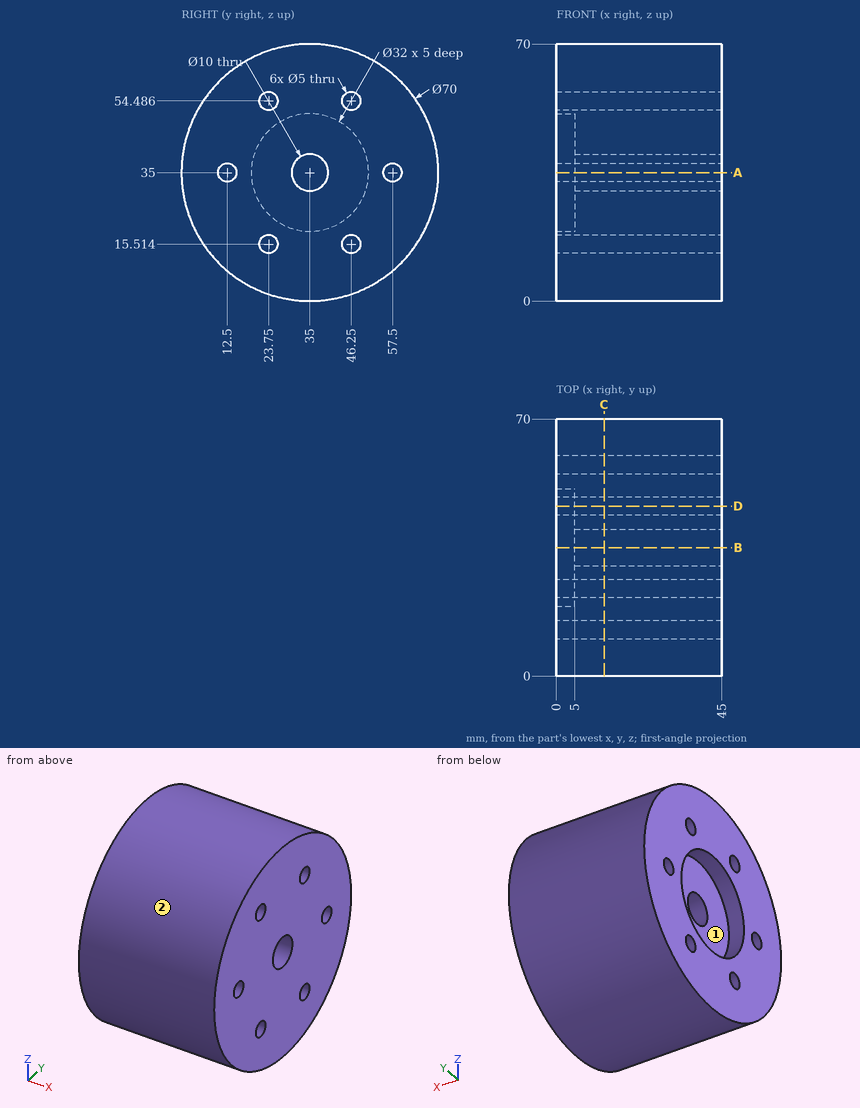
Can you work these out from the drawing? Everything is in mm from the part's minimum corner. A direction names the side the tool comes from. Give positions to 0.01 mm unless a question says otherwise; leave off trailing zeros. Loops run counter-clockwise (first coordinate to the right, second up) from the corner with the lowest first, then second, coordinate; pieces in that order, holes last. Notation, with made-up numbers: (7, 39.5) - (44, 39.5) arc R12 cw to (44, 49.5) - close; hole circle Ø1 at (19.25, -31). An arc over 180 degrees is marked (long way). Use one line per item in the form item = value.
1. I'm going to push flat-ended pins straight in: pin 1 Ø4.5 at (y, z) = (23.75, 54.49) entering from -X; pin 2 Ø1 at (y, z) = (25.5, 46.5) entering from -X; pin 3 Ø6 at (x, y) = (5.5, 59.5) entering from -Z; pin 4 Ø1 at (x, z) = (5.5, 40) entering from +Y. Where does each tip first touch, or does it pass through?
Response values:
pin_1 = through
pin_2 = 5
pin_3 = 7.38
pin_4 = 69.71
2. I want a section at D-D (y = 46.25). Please give me the cut outline in (x, z) (1 decimal), and give its area (3 significant figures).
Response values:
outline = (0, 1.9) - (45, 1.9) - (45, 13) - (0, 13) - close; (0, 18) - (45, 18) - (45, 52) - (0, 52) - (0, 46.4) - (5, 46.4) - (5, 23.6) - (0, 23.6) - close; (0, 57) - (45, 57) - (45, 68.1) - (0, 68.1) - close
area = 2,420 mm²
3. I want a section at C-C (x = 13). Give the number of separate pieces and of enclosed holes in the cut face, and give its area (3 significant figures).
Response values:
separate_pieces = 1
enclosed_holes = 7
area = 3,650 mm²
4. I need wall thicknesses on probe 1 along Y at (x, z) = (24, 35); probe 2 along Z at (x, y) = (9, 23); probe 3 along Z at (x, y) = (19, 23.5). Which ranges of each line are inside material? Lowest first, please.
Response values:
probe_1 = 0 to 10, 15 to 30, 40 to 55, 60 to 70
probe_2 = 2.12 to 13.13, 17.9 to 52.1, 56.87 to 67.88
probe_3 = 1.94 to 13.03, 18 to 52, 56.97 to 68.06
5. I want a section at B-B (y = 35). Please give me the cut outline in (x, z), and give its area (3 significant figures).
Response values:
outline = (0, 0) - (45, 0) - (45, 30) - (5, 30) - (5, 19) - (0, 19) - close; (0, 51) - (5, 51) - (5, 40) - (45, 40) - (45, 70) - (0, 70) - close
area = 2,590 mm²
6. On a 3-axis mill with a long thin cutter (end or side, diameter ignored), from which of +Z, -Z, +X, -X, +Y, -Y can I reach the whole of each face in a straight line? I mean the marked faces 1 and 2. Say none if no direction works.
Response values:
face_1 = -X
face_2 = +X, -X
7. I want a section at A-A (z = 35). Please give me the cut outline in (x, y).
Response values:
outline = (0, 0) - (45, 0) - (45, 10) - (0, 10) - close; (0, 15) - (45, 15) - (45, 30) - (5, 30) - (5, 19) - (0, 19) - close; (0, 51) - (5, 51) - (5, 40) - (45, 40) - (45, 55) - (0, 55) - close; (0, 60) - (45, 60) - (45, 70) - (0, 70) - close
